Design review of the part built by this model. Coordinates are the model's own, in mm. A direction names the side the tool comes from. Coordinates: 2 decimals unless noted, no trailing zeros. Write each loop counter-clockwise with the first axis right and the second up, starting at its lowest first coordinate (ties: lowest second). Pieces come first, ordered by that corner, then holes.
Q1. Take a section at B-B (y = 14). Give the boundary of the cut face in (x, z).
Q2. Machinability: for faces 1 (the flat face through (8, -2, 43)), 2 (the cylindrical face through (3.324, -0.855, 0.986)), 3 (the flat face through (28.737, -11, 23)), which of the approach directions +Z, -Z, +X, -X, +Y, -Y give a long, thin tool a straight path to every point of the face, cutting with its end or side? Answer none if there is none.
Q3. Insertion check: pin 1 (6 mm diameter, centred on x = -4.16, y = -24.9, fed in from -Z); pin 2 (9.5 mm diameter, centred on x = 8.24, y = -2.4, fed in from +Z); pin 3 (1 mm diameter, centred on x = 20.5, y = 13, fed in from -Z); pin 4 (3 mm diameter, centred on x = 8.5, y = 0, fed in from -Z). Each pin has a flat end and moves straight along its axis. Give the tip position at first contact, or say it passes through.
Q4. Mouldability with a two-part tool opening along Z and no side actions: class faces 4 (the cylindrical face through (8.55, 17.59, 40.72)), 5 (the flat face through (8, 22.098, 22)), 6 (the cylindrical face through (29.75, 13.5, 21.67)) as pulls with the +Z half, pulls with the -Z half, needs draft (parallel to the pull), parting line crosses it, or undercut.
Q5. Take a section at C-C (x = 2). Give the boundary of the cut face in (y, z) (3 decimals).
Q6. Take a section at A-A (z = 22.5). State how many separate pieces and enclosed holes the cut face has, and give its area (3 significant figures).
Q7. For probe 1 along Y at (x, z) = (30.05, 22.5); probe 2 along Y at (x, z) = (2, 22.5); probe 3 along Y at (x, z) = (30, 22), list the stretches that pass through material, from the lowest coordinate up.
Q8. Take a section at D-D (y = -4.5). Give the boundary of the cut face in (x, z), and give its area (3 significant figures).
```python
from build123d import *

# Parameters (mm, degrees)
SKETCH1_W           = 45
SKETCH1_H           = 50
BOSS_EXTRUDE1_DEPTH = 45
SKETCH2_R           = 5.2
CUT_EXTRUDE1_DEPTH  = 45
SKETCH9_R           = 5.15
CUT_EXTRUDE6_DEPTH  = 2
SKETCH10_R          = 5.15
CUT_EXTRUDE7_DEPTH  = 2
SKETCH12_R          = 18.375
CUT_EXTRUDE8_DEPTH  = 45
SKETCH13_W          = 45
SKETCH13_H          = 6.66747138
CUT_EXTRUDE9_DEPTH  = 46
SKETCH14_W          = 45
SKETCH14_H          = 6.66747138
BOSS_EXTRUDE2_DEPTH = 45
SKETCH15_R          = 18.375
CUT_EXTRUDE10_DEPTH = 45
FILLET1_R           = 15
SKETCH16_R          = 18.375
BOSS_EXTRUDE3_DEPTH = 2
SKETCH17_R          = 11.5
CUT_EXTRUDE11_DEPTH = 2
SKETCH18_R          = 1.8
CUT_EXTRUDE12_DEPTH = 2
BOSS_EXTRUDE4_DEPTH = 45


with BuildPart() as part:
    # Sketch1 → Boss-Extrude1 (new body)
    with BuildSketch(Plane.XY):
        with Locations((8.236607143, -2.901785714)):
            Rectangle(SKETCH1_W, SKETCH1_H)
    extrude(amount=BOSS_EXTRUDE1_DEPTH)

    # Sketch2 → Cut-Extrude1 (cut)
    with BuildSketch(Plane.XY.offset(45)):
        with Locations((-4.163392857, -24.901785714)):
            Circle(SKETCH2_R)
        with Locations((20.636607143, -24.901785714)):
            Circle(SKETCH2_R)
    extrude(amount=-CUT_EXTRUDE1_DEPTH, mode=Mode.SUBTRACT)

    # Sketch9 → Cut-Extrude6 (cut)
    with BuildSketch(Plane.XY.offset(45)):
        with Locations((8.236607143, -2.401785714)):
            Circle(SKETCH9_R)
    extrude(amount=-CUT_EXTRUDE6_DEPTH, mode=Mode.SUBTRACT)

    # Sketch10 → Cut-Extrude7 (cut)
    with BuildSketch(Plane(origin=(0, 0, 0), x_dir=(-1, 0, 0), z_dir=(0, 0, -1))):
        with Locations((-8.236607143, -2.401785714)):
            Circle(SKETCH10_R)
    extrude(amount=-CUT_EXTRUDE7_DEPTH, mode=Mode.SUBTRACT)

    # Sketch12 → Cut-Extrude8 (cut)
    with BuildSketch(Plane.ZY.offset(14.263392857)):
        with Locations((22.5, 1.098214286)):
            Circle(SKETCH12_R)
    extrude(amount=-CUT_EXTRUDE8_DEPTH, mode=Mode.SUBTRACT)

    # Sketch13 → Cut-Extrude9 (cut)
    with BuildSketch(Plane.ZY.offset(14.263392857)):
        with Locations((22.5, 18.764478596)):
            Rectangle(SKETCH13_W, SKETCH13_H)
    extrude(amount=-CUT_EXTRUDE9_DEPTH, mode=Mode.SUBTRACT)

    # Sketch14 → Boss-Extrude2 (add)
    with BuildSketch(Plane.ZY.offset(14.263392857)):
        with Locations((22.5, 18.764478596)):
            Rectangle(SKETCH14_W, SKETCH14_H)
    extrude(amount=-BOSS_EXTRUDE2_DEPTH)

    # Sketch15 → Cut-Extrude10 (cut)
    with BuildSketch(Plane.ZY.offset(14.263392857)):
        with Locations((22.5, 1.098214286)):
            Circle(SKETCH15_R)
    extrude(amount=-CUT_EXTRUDE10_DEPTH, mode=Mode.SUBTRACT)

    # Fillet1
    fillet1_edges = [part.edges().sort_by_distance(p)[0] for p in [
        (8.236607143, 22.098214286, 0),
        (8.236607143, 22.098214286, 45),
    ]]
    fillet(fillet1_edges, radius=FILLET1_R)

    # Sketch16 → Boss-Extrude3 (add)
    with BuildSketch(Plane(origin=(30.736607143, 0, 0), x_dir=(0, 0, -1), z_dir=(1, 0, 0))):
        with Locations((-22.5, 1.098214286)):
            Circle(SKETCH16_R)
    extrude(amount=-BOSS_EXTRUDE3_DEPTH)

    # Sketch17 → Cut-Extrude11 (cut)
    with BuildSketch(Plane(origin=(30.736607143, 0, 0), x_dir=(0, 0, -1), z_dir=(1, 0, 0))):
        with Locations((-22.5, 1.098214286)):
            Circle(SKETCH17_R)
    extrude(amount=-CUT_EXTRUDE11_DEPTH, mode=Mode.SUBTRACT)

    # Sketch18 → Cut-Extrude12 (cut)
    with BuildSketch(Plane(origin=(30.736607143, 0, 0), x_dir=(0, 0, -1), z_dir=(1, 0, 0))):
        with Locations((-22.5, 15.098214286)):
            Circle(SKETCH18_R)
    extrude(amount=-CUT_EXTRUDE12_DEPTH, mode=Mode.SUBTRACT)

    # Sketch19 → Boss-Extrude4 (add)
    with BuildSketch(Plane.XY.offset(45)):
        with BuildLine():
            Line((0.043119335, -27.87293956), (0.02274465, -27.901785714))
            Line((0.02274465, -27.901785714), (0.083959259, -27.901785714))
            ThreePointArc((0.083959259, -27.901785714), (-4.163392857, -19.701785714), (-8.410744973, -27.901785714))
            Line((-8.410744973, -27.901785714), (-8.286832824, -27.901785714))
            Line((-8.286832824, -27.901785714), (-8.369905049, -27.87293956))
            ThreePointArc((-8.369905049, -27.87293956), (-4.163392857, -19.751785714), (0.043119335, -27.87293956))
        make_face()
        with BuildLine():
            Line((16.430094951, -27.87293956), (16.516624547, -27.901785714))
            Line((16.516624547, -27.901785714), (16.389255027, -27.901785714))
            ThreePointArc((16.389255027, -27.901785714), (20.636607143, -19.701785714), (24.883959259, -27.901785714))
            Line((24.883959259, -27.901785714), (24.82274465, -27.901785714))
            Line((24.82274465, -27.901785714), (24.843119335, -27.87293956))
            ThreePointArc((24.843119335, -27.87293956), (20.636607143, -19.751785714), (16.430094951, -27.87293956))
        make_face()
    extrude(amount=-BOSS_EXTRUDE4_DEPTH)


solid = part.part
```
Response:
1. outline: (-14.26, 1.68) - (30.74, 1.68) - (30.74, 21.07) - (28.74, 21.07) - (28.74, 9.42) - (-14.26, 9.42) - close; (-14.26, 35.58) - (28.74, 35.58) - (28.74, 23.93) - (30.74, 23.93) - (30.74, 43.32) - (-14.26, 43.32) - close
2. face 1: +Z
2. face 2: -Z
2. face 3: -X
3. pin 1: passes through
3. pin 2: stops at z = 43
3. pin 3: stops at z = 1.01
3. pin 4: stops at z = 2
4. face 4: pulls with the +Z half
4. face 5: needs draft
4. face 6: undercut
5. outline: (-27.902, 0) - (7.098, 0) arc R15 ccw to (22.098, 15) - (22.098, 30) arc R15 ccw to (7.098, 45) - (-27.902, 45) - close; hole circle Ø36.75 at (1.098, 22.5)
6. separate pieces: 3
6. enclosed holes: 0
6. area: 475 mm2
7. probe 1: y = -27.9 to -10.4, 12.6 to 13.3, 16.9 to 22.1
7. probe 2: y = -27.9 to -17.28, 19.47 to 22.1
7. probe 3: y = -27.9 to -10.39, 12.59 to 13.37, 16.83 to 22.1
8. outline: (-14.26, 0) - (3.53, 0) - (3.53, 2) - (12.94, 2) - (12.94, 0) - (30.74, 0) - (30.74, 12.45) - (28.74, 12.45) - (28.74, 5) - (-14.26, 5) - close; (-14.26, 40) - (28.74, 40) - (28.74, 32.55) - (30.74, 32.55) - (30.74, 45) - (12.94, 45) - (12.94, 43) - (3.53, 43) - (3.53, 45) - (-14.26, 45) - close
8. area: 442 mm2
